from build123d import *

# Parameters (mm, degrees)
SKETCH2_R           = 60
BOSS_EXTRUDE1_DEPTH = 120
SKETCH4_W           = 7.5
SKETCH4_H           = 100
SKETCH4_W_2         = 15.517169794
SKETCH4_W_3         = 15
CUT_EXTRUDE1_DEPTH  = 60


with BuildPart() as part:
    # Sketch2 → Boss-Extrude1 (new body)
    with BuildSketch(Plane(origin=(0, 0, 0), x_dir=(1, 0, 0), z_dir=(0, 1, 0))):
        with Locations(Location((0, 0, 0), (0, 0, 270))):
            Circle(SKETCH2_R)
    extrude(amount=BOSS_EXTRUDE1_DEPTH)

    # Sketch4 → Cut-Extrude1 (cut, symmetric)
    with BuildSketch(Plane.XY):
        with Locations((-56.25, 70)):
            Rectangle(SKETCH4_W, SKETCH4_H)
        with Locations((-40.258584897, 70)):
            Rectangle(SKETCH4_W_2, SKETCH4_H)
        with Locations((-20, 70)):
            Rectangle(SKETCH4_W_3, SKETCH4_H)
        with Locations((0, 70)):
            Rectangle(SKETCH4_W_3, SKETCH4_H)
        with Locations((20, 70)):
            Rectangle(SKETCH4_W_3, SKETCH4_H)
        with Locations((40.258584897, 70)):
            Rectangle(SKETCH4_W_2, SKETCH4_H)
        with Locations((56.25, 70)):
            Rectangle(SKETCH4_W, SKETCH4_H)
    extrude(amount=CUT_EXTRUDE1_DEPTH, both=True, mode=Mode.SUBTRACT)


solid = part.part
Can you work these out from the model? Positions are in its coordinate system, mm. A direction names the side the tool comes from. Round coordinates to 2 decimals unless told otherwise and drop trailing zeros. Write each loop counter-clockwise with the first axis right and the second up, starting at its lowest first coordinate (ties: lowest second). Pieces come first, ordered by that corner, then holes. Notation, with made-up numbers: (24.25, -9.5) -> (44.25, -9.5) arc R28 ccw to (44.25, 23.5) -> close; hole circle Ø7 at (20, -4.75). An arc over 180 degrees is marked (long way). One line per question, with ' | ' between items. Start each with the question number.
1) Suppose I cut it at D-D on z = -18. Write out the boundary of the cut face in (x, y), then the cut area to 3 significant figures.
2) Suppose I cut it at B-B on z = 0. Write out the boundary of the cut face in (x, y), then the cut area to 3 significant figures.
3) Suppose I cut it at A-A on y = 108.5. Write out the boundary of the cut face in (x, z), then the cut area to 3 significant figures.
4) I need wall thicknesses on line 1 (X direction, y = 72.5, z = 1); line 2 (X direction, y = 38, z = -43); line 3 (X direction, y = 24, z = -35.5). Which ranges of each line are inside material? Lowest first, please. Write a range as [from, to].
5) If we mould it in two halves opening along X, with no side actions, what happens to faces 4 (the flat face through (-20, 20, -1)), 5 (the flat face through (52.5, 69, 0)), 6 (the flat face through (-48.017, 69, -1)), 7 (the flat face through (1, 0, -1))? For each: released by +X, released by -X, zero draft, split by the parting line, or undercut.
6) Suppose I cut it at C-C on x = -16. Write out the boundary of the cut face in (y, z).
7) I'm going to push flat-ended pins straight in: P1, Ø12, axis at x = 0, y = 56, coming from the +Z side; P2, Ø2, axis at x = 57.5, z = 14, coming from the +Y side; P3, Ø1, axis at y = 46, z = -2, coming from the -X side; P4, Ø21.5, axis at y = 62, z = -6, coming from the +X side. Where does each tip first touch, or does it pass through?
8) On a 3-axis mill with a long thin cutter (end or side, diameter ignored), from which of +Z, -Z, +X, -X, +Y, -Y can I reach the whole of each face in a straight line? I mean faces 1 (the flat face through (-55, 20, 0)), 2 (the flat face through (27.5, 69, -1)), 3 (the flat face through (55, 20, 0)). Say none if no direction works.
Return value:
1) outline: (-57.24, 0) -> (57.24, 0) -> (57.24, 20) -> (52.5, 20) -> (52.5, 120) -> (48.02, 120) -> (48.02, 20) -> (32.5, 20) -> (32.5, 120) -> (27.5, 120) -> (27.5, 20) -> (12.5, 20) -> (12.5, 120) -> (7.5, 120) -> (7.5, 20) -> (-7.5, 20) -> (-7.5, 120) -> (-12.5, 120) -> (-12.5, 20) -> (-27.5, 20) -> (-27.5, 120) -> (-32.5, 120) -> (-32.5, 20) -> (-48.02, 20) -> (-48.02, 120) -> (-52.5, 120) -> (-52.5, 20) -> (-57.24, 20) -> close | area: 5,190 mm2
2) outline: (-60, 0) -> (60, 0) -> (60, 20) -> (52.5, 20) -> (52.5, 120) -> (48.02, 120) -> (48.02, 20) -> (32.5, 20) -> (32.5, 120) -> (27.5, 120) -> (27.5, 20) -> (12.5, 20) -> (12.5, 120) -> (7.5, 120) -> (7.5, 20) -> (-7.5, 20) -> (-7.5, 120) -> (-12.5, 120) -> (-12.5, 20) -> (-27.5, 20) -> (-27.5, 120) -> (-32.5, 120) -> (-32.5, 20) -> (-48.02, 20) -> (-48.02, 120) -> (-52.5, 120) -> (-52.5, 20) -> (-60, 20) -> close | area: 5,300 mm2
3) outline: (-52.5, -29.05) arc R60 ccw to (-48.02, -35.98) -> (-48.02, 35.98) arc R60 ccw to (-52.5, 29.05) -> close; (-32.5, -50.44) arc R60 ccw to (-27.5, -53.33) -> (-27.5, 53.33) arc R60 ccw to (-32.5, 50.44) -> close; (-12.5, -58.68) arc R60 ccw to (-7.5, -59.53) -> (-7.5, 59.53) arc R60 ccw to (-12.5, 58.68) -> close; (7.5, -59.53) arc R60 ccw to (12.5, -58.68) -> (12.5, 58.68) arc R60 ccw to (7.5, 59.53) -> close; (27.5, -53.33) arc R60 ccw to (32.5, -50.44) -> (32.5, 50.44) arc R60 ccw to (27.5, 53.33) -> close; (48.02, -35.98) arc R60 ccw to (52.5, -29.05) -> (52.5, 29.05) arc R60 ccw to (48.02, 35.98) -> close | area: 2,810 mm2
4) line 1: x = [-52.5, -48.02], [-32.5, -27.5], [-12.5, -7.5], [7.5, 12.5], [27.5, 32.5], [48.02, 52.5] | line 2: x = [-32.5, -27.5], [-12.5, -7.5], [7.5, 12.5], [27.5, 32.5] | line 3: x = [-48.37, -48.02], [-32.5, -27.5], [-12.5, -7.5], [7.5, 12.5], [27.5, 32.5], [48.02, 48.37]
5) face 4: undercut | face 5: released by +X | face 6: undercut | face 7: zero draft
6) outline: (0, -57.83) -> (20, -57.83) -> (20, 57.83) -> (0, 57.83) -> close
7) P1: passes through | P2: stops at y = 20 | P3: stops at x = -52.5 | P4: stops at x = 52.5
8) face 1: +Z, -Z, -X, +Y | face 2: +Z, -Z, +Y | face 3: +Z, -Z, +X, +Y
